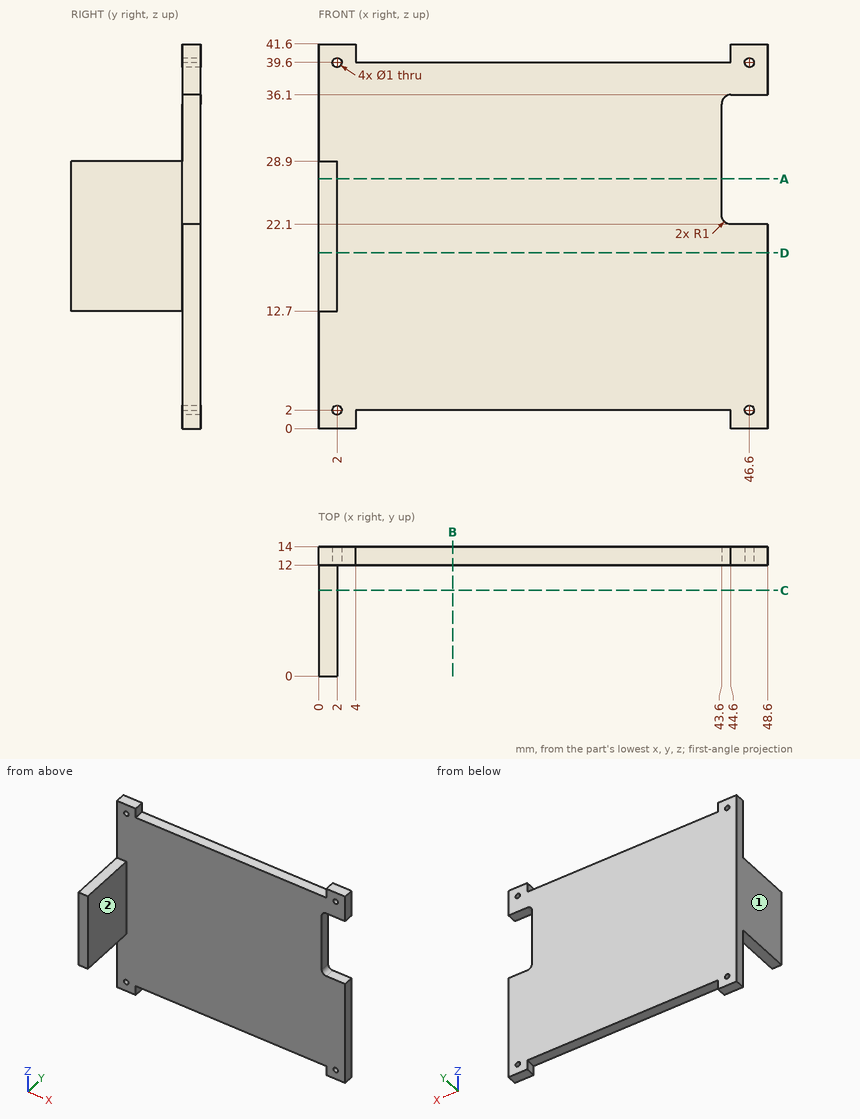
Here's the drawing with two shaded views (mm, measured from the low corner). I have some questions. A direction names the side the tool comes from. Coordinates: 2 decimals unless noted, no trailing zeros. Write each loop counter-clockwise with the first axis right and the second up, starting at its lowest first coordinate (ties: lowest second). Pieces come first, ordered by that corner, then holes. Notation, with made-up numbers: (53.5, 73.5) -> (92.5, 73.5) arc R11 ccw to (92.5, 89.5) -> close; hole circle Ø6 at (-13, 12). An arc over 180 degrees is marked (long way). Write item = value, one per line. Start each with the question number.
(1) I want a section at D-D (z = 19). Please give me the cut outline in (x, y), plus the area to 3 significant figures.
(2) Which directions (+Z, -Z, +X, -X, +Y, -Y) give clear straight access to the entire face, cutting with the end or side of a thin tool? Please do the marked faces 1 and 2.
(3) I want a section at A-A (z = 27). Please give me the cut outline in (x, y).
(4) Will these pins go through, and if not, where does the flat tip stop? pin 1 (0.6 mm diameter, centred on x = 28, y = 12.5, fed in from +Z); pin 2 (5 mm diameter, centred on x = 12.5, z = 35.5, fed in from -Y); pin 3 (1.6 mm diameter, centred on x = 1, y = 6, fed in from -Z); pin 4 (1 mm diameter, centred on x = 47, y = 13, fed in from -Z).
(5) I need wall thicknesses on line 1 (Z direction, x = 2, y = 12.85); line 2 (Z direction, x = 46.6, y = 13.55); line 3 (X direction, y = 12.75, z = 25). Which ranges of each line are inside material? Lowest first, please. Write a range as [from, to].
(6) I want a section at B-B (x = 14.5). Please give me the cut outline in (y, z), plus the area to 3 significant figures.
(7) I want a section at C-C (y = 9.25). Please give me the cut outline in (x, z), plus the area to 3 significant figures.
Result set:
q1.outline = (0, 0) -> (2, 0) -> (2, 12) -> (48.6, 12) -> (48.6, 14) -> (0, 14) -> close
q1.area = 121 mm2
q2.face_1 = +Z, -Z, -X, +Y, -Y
q2.face_2 = +Z, -Z, +X, -Y
q3.outline = (0, 0) -> (2, 0) -> (2, 12) -> (43.6, 12) -> (43.6, 14) -> (0, 14) -> close
q4.pin_1 = 39.6
q4.pin_2 = 12
q4.pin_3 = 12.7
q4.pin_4 = 0
q5.line_1 = [0, 1.5], [2.5, 39.1], [40.1, 41.6]
q5.line_2 = [0, 1.5], [2.5, 22.1], [36.1, 39.1], [40.1, 41.6]
q5.line_3 = [0, 43.6]
q6.outline = (12, 2) -> (14, 2) -> (14, 39.6) -> (12, 39.6) -> close
q6.area = 75.2 mm2
q7.outline = (0, 12.7) -> (2, 12.7) -> (2, 28.9) -> (0, 28.9) -> close
q7.area = 32.4 mm2
